Here's how the part is built. I have some questions about the finished solid (model axes, mm). Face numbers are marked on the shaded views. A direction names the side the tool comes from. Coordinates: 2 decimals unless noted, no trailing zeros. Write each loop counter-clockwise with the first axis right and the second up, starting at its lowest first coordinate (ties: lowest second). Pieces come first, ordered by that corner, then holes.
(1) Thinking about a two-plate mould opening in Y: for the marked faces 1, 2 and 3, which applies, released by +Y, released by -Y, zero draft, split by the parting line, or undercut?
(2) Imagine slicing it at B-B, the plane y = 393.7. State how many separate pieces and enclosed holes the cut face has, plus the area to 3 significant figures.
(3) For pin 1 Ø4 at (y, z) = (311, 165.5) entering from +X; pin 2 Ø22.5 at (x, y) = (17.5, 849) entering from -Z; pin 3 Ø5.5 at (x, y) = (649.5, 392) entering from -Z; pin 4 Ø7.5 at (y, z) = (480.5, 101) entering from +X, each with a flat end and sliding along its axis, tell me the tip position at first contact or that it passes through.
(4) Imagine slicing it at C-C, the plane x = 12.7. List the corners of the cut face in (y, z) for me, plus the area to 3 significant figures.
(5) Please list where these lines run through material, in increasing order: probe 1 along Y at (x, z) = (71.5, 169); probe 2 along Y at (x, z) = (12, 9); probe 3 along X at (y, z) = (850.9, 192) (3 decimals).
(6) Imagine slicing it at A-A, the plane x = 368.3. List the corners of the cut face in (y, z) for me (3 decimals), plus the area to 3 significant figures.
(7) Which directions (+Z, -Z, +X, -X, +Y, -Y) give clear straight access to the entire face, cutting with the end or side of a thin tool? Please do the marked faces 4 and 5.
(8) Imagine slicing it at D-D, the plane y = 283. List the corners of the cut face in (x, z) for me, plus the area to 3 significant figures.
```python
from build123d import *

# Parameters (mm, degrees)
F0_W      = 101.6
F0_H      = 368.3
F0_W_2    = 203.2
F0_H_2    = 25.4
F1_DEPTH  = 203.2
F2_R      = 10.16
F2_R_2    = 9.525
F3_DEPTH  = 12.7
F4_DEPTH  = 203.2
F5_DEPTH  = 31.75
F6_W      = 50.8
F6_H      = 76.2
F7_DEPTH  = 25.4
F9_DEPTH  = 25.4
F11_DEPTH = 2540
F13_DEPTH = 25.4
F15_DEPTH = 25.4
F16_W     = 88.9
F16_H     = 76.2
F17_DEPTH = 25.4
F16_W_2   = 101.6
F16_H_2   = 101.6
F18_DEPTH = 25.4
F19_R     = 9.525
F20_DEPTH = 19.05


# Not quite as in the source:
# - a feature names something its author has since deleted; it is built from what else it names


with BuildPart() as f1:
    # F0 (on Top) → F1 (new body)
    with BuildSketch(Plane.XY):
        Polygon((0, 863.6), (0, 0), (381, 0), (381, 381), (660.4, 381), (660.4, 406.4), (660.4, 838.2), (660.4, 863.6), align=None)
        Polygon((406.4, 838.2), (635, 838.2), (635, 406.4), (355.6, 406.4), (355.6, 25.4), (25.4, 25.4), (25.4, 38.7719720602), (25.4, 330.2), (25.4, 355.6), (25.4, 469.9), (25.4, 495.3), (25.4, 838.2), (304.8, 838.2), align=None, mode=Mode.SUBTRACT)
        with Locations((355.6, 654.05)):
            Rectangle(F0_W, F0_H)
        Polygon((254, 355.6), (25.4, 355.6), (25.4, 330.2), (279.4, 330.2), (279.4, 355.6), (279.4, 381), (254, 381), align=None)
        with Locations((127, 482.6)):
            Rectangle(F0_W_2, F0_H_2)
    extrude(amount=F1_DEPTH)

    # F2 (on face) → F3 (cut)
    with BuildSketch(Plane(origin=(0, 0, 0), x_dir=(1, 0, 0), z_dir=(0, 0, -1))):
        with Locations((12.7, -850.9)):
            Circle(F2_R)
        with Locations((12.7, -12.7)):
            Circle(F2_R)
        with Locations((368.3, -12.7)):
            Circle(F2_R)
        with Locations((647.7, -850.9)):
            Circle(F2_R_2)
        with Locations((368.3, -393.7)):
            Circle(F2_R_2)
        with Locations((647.7, -393.7)):
            Circle(F2_R_2)
    extrude(amount=-F3_DEPTH, mode=Mode.SUBTRACT)

    # F4 (add): faces of the model
    f4_faces = [f1.faces().sort_by_distance(p)[0] for p in [
        (12.7, 12.7, 12.7),
        (368.3, 12.7, 12.7),
        (12.7, 850.9, 12.7),
    ]]
    extrude(f4_faces, amount=-F4_DEPTH)

    # F5 (cut): faces of the model
    f5_faces = [f1.faces().sort_by_distance(p)[0] for p in [
        (12.7, 850.9, 215.9),
        (368.3, 12.7, 215.9),
        (12.7, 12.7, 215.9),
    ]]
    extrude(f5_faces, amount=-F5_DEPTH, mode=Mode.SUBTRACT)

    # F6 (on face) → F7 (cut)
    with BuildSketch(Plane.XZ):
        with Locations((120.65, 139.7)):
            Rectangle(F6_W, F6_H)
        with Locations((69.85, 139.7)):
            Rectangle(F6_W, F6_H)
        Polygon((234.95, 177.8), (234.95, 101.6), (336.55, 101.6), (336.55, 177.8), (285.75, 177.8), align=None)
    extrude(amount=-F7_DEPTH, mode=Mode.SUBTRACT)

    # F8 (on face) → F9 (cut)
    with BuildSketch(Plane.YZ.offset(381)):
        Polygon((165.1, 76.2), (190.5, 76.2), (266.7, 76.2), (266.7, 177.8), (165.1, 177.8), align=None)
    extrude(amount=-F9_DEPTH, mode=Mode.SUBTRACT)

    # F10 (on face) → F11 (cut)
    with BuildSketch(Plane.XZ.offset(-381)):
        Polygon((482.6, 76.2), (533.4, 76.2), (584.2, 76.2), (584.2, 177.8), (482.6, 177.8), align=None)
    extrude(amount=-F11_DEPTH, mode=Mode.SUBTRACT)

    # F12 (on face) → F13 (cut)
    with BuildSketch(Plane.YZ.offset(660.4)):
        Polygon((450.85, 76.2), (501.65, 76.2), (552.45, 76.2), (552.45, 177.8), (450.85, 177.8), align=None)
        Polygon((793.75, 177.8), (692.15, 177.8), (692.15, 76.2), (742.95, 76.2), (793.75, 76.2), align=None)
    extrude(amount=-F13_DEPTH, mode=Mode.SUBTRACT)

    # F14 (on face) → F15 (cut)
    with BuildSketch(Plane(origin=(0, 863.6, 0), x_dir=(-1, 0, 0), z_dir=(0, 1, 0))):
        Polygon((-206.375, 177.8), (-257.175, 177.8), (-307.975, 177.8), (-307.975, 76.2), (-206.375, 76.2), align=None)
    extrude(amount=-F15_DEPTH, mode=Mode.SUBTRACT)

    # F16 (on face) → F17 (cut)
    with BuildSketch(Plane(origin=(0, 0, 0), x_dir=(0, -1, 0), z_dir=(-1, 0, 0))):
        with Locations((-412.75, 139.7)):
            Rectangle(F16_W, F16_H)
    extrude(amount=-F17_DEPTH, mode=Mode.SUBTRACT)

    # F16 (on face) → F18 (cut)
    with BuildSketch(Plane(origin=(0, 0, 0), x_dir=(0, -1, 0), z_dir=(-1, 0, 0))):
        with Locations((-412.75, 139.7)):
            Rectangle(F16_W, F16_H)
        with Locations((-615.95, 127)):
            Rectangle(F16_W_2, F16_H_2)
    extrude(amount=-F18_DEPTH, mode=Mode.SUBTRACT)

    # F19 (on face) → F20 (cut)
    with BuildSketch(Plane.XY.offset(203.2)):
        with Locations((368.3, 393.7)):
            Circle(F19_R)
        with Locations((647.7, 393.7)):
            Circle(F19_R)
        with Locations((647.7, 850.9)):
            Circle(F19_R)
    extrude(amount=-F20_DEPTH, mode=Mode.SUBTRACT)


solid = f1.part
```
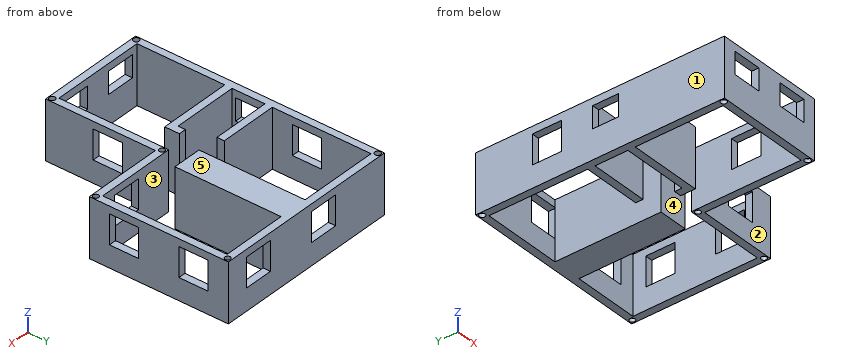
Recorded:
1. face 1: zero draft
1. face 2: released by -Y
1. face 3: undercut
2. separate pieces: 3
2. enclosed holes: 1
2. area: 53,600 mm2
3. pin 1: stops at x = 381
3. pin 2: stops at z = 0
3. pin 3: stops at z = 12.7
3. pin 4: stops at x = 406.4
4. outline: (0, 0) - (2.54, 0) - (2.54, 12.7) - (22.86, 12.7) - (22.86, 0) - (840.74, 0) - (840.74, 12.7) - (861.06, 12.7) - (861.06, 0) - (863.6, 0) - (863.6, 203.2) - (861.06, 203.2) - (861.06, 184.15) - (840.74, 184.15) - (840.74, 203.2) - (22.86, 203.2) - (22.86, 184.15) - (2.54, 184.15) - (2.54, 203.2) - (0, 203.2) - close; hole (368.3, 101.6) - (457.2, 101.6) - (457.2, 177.8) - (368.3, 177.8) - close; hole (565.15, 76.2) - (666.75, 76.2) - (666.75, 177.8) - (565.15, 177.8) - close
4. area: 157,000 mm2
5. probe 1: y = 330.2 to 355.6, 469.9 to 495.3, 838.2 to 863.6
5. probe 2: y = 0 to 2.56, 22.84 to 840.76, 861.04 to 863.6
5. probe 3: x = 0 to 2.54, 22.86 to 638.175, 657.225 to 660.4
6. outline: (0, 0) - (2.54, 0) - (2.54, 12.7) - (22.86, 12.7) - (22.86, 0) - (384.175, 0) - (384.175, 12.7) - (403.225, 12.7) - (403.225, 0) - (406.4, 0) - (406.4, 203.2) - (403.225, 203.2) - (403.225, 184.15) - (384.175, 184.15) - (384.175, 203.2) - (22.86, 203.2) - (22.86, 184.15) - (2.54, 184.15) - (2.54, 203.2) - (0, 203.2) - close; (469.9, 0) - (863.6, 0) - (863.6, 203.2) - (469.9, 203.2) - close; hole (165.1, 76.2) - (266.7, 76.2) - (266.7, 177.8) - (165.1, 177.8) - close
6. area: 151,000 mm2
7. face 4: +Z, -Z
7. face 5: +Z, +X, -X, +Y, -Y
8. outline: (0, 0) - (25.4, 0) - (25.4, 203.2) - (0, 203.2) - close; (355.6, 0) - (381, 0) - (381, 203.2) - (355.6, 203.2) - close
8. area: 10,300 mm2
